Here's how the part is built. I have some questions about the finished solid (model axes, mm). A direction names the side the tool comes from. Round coordinates to 2 decimals unless told otherwise and drop trailing zeros. Order: outer loops, then holes, each group sorted by start corner. A loop starts at its lowest first (then second) coordinate and runs counter-clockwise, first axis right, second up. Notation, with made-up numbers: (72, 52) - (114, 52) arc R14 cw to (114, 72) - close; hole circle Ø1 at (-24, 66). An arc over 180 degrees is marked (long way). Answer as a JSON object with one key per item and string values.
```python
from build123d import *

# Parameters (mm, degrees)
SKETCH1_R           = 7.874
BOSS_EXTRUDE1_DEPTH = 65.024
SKETCH2_R           = 12.7
BOSS_EXTRUDE2_DEPTH = 6.35
CHAMFER1_SIZE       = 2.54


with BuildPart() as part:
    # Sketch1 → Boss-Extrude1 (new body)
    with BuildSketch(Plane.XY):
        Circle(SKETCH1_R)
    extrude(amount=-BOSS_EXTRUDE1_DEPTH)

    # Sketch2 → Boss-Extrude2 (add)
    with BuildSketch(Plane.XY):
        Circle(SKETCH2_R)
    extrude(amount=-BOSS_EXTRUDE2_DEPTH)

    # Chamfer1
    chamfer1_edges = [part.edges().sort_by_distance(p)[0] for p in [
        (-12.7, 0, 0),
    ]]
    chamfer(chamfer1_edges, length=CHAMFER1_SIZE)


solid = part.part
```
1. Imagine slicing it at C-C (z = -50). List the corners of the cut face in (x, y) for me.
Responses:
{"outline": "circle Ø15.75 at (0, 0)"}
2. If I drill on L1, parallel to Z at x = -9.5, y = -5; L2, parallel to X at y = 2, z = -44.5; L3, parallel to Y at x = 0.75, z = -12.5, over which ranges is the centre line in solid material (lowest first)? Write a range as [from, to].
Responses:
{"L1": "[-6.35, -0.58]", "L2": "[-7.62, 7.62]", "L3": "[-7.84, 7.84]"}
3. Imagine slicing it at A-A (x = 0). List the corners of the cut face in (y, z) for me.
Responses:
{"outline": "(-12.7, -6.35) - (-7.87, -6.35) - (-7.87, -65.02) - (7.87, -65.02) - (7.87, -6.35) - (12.7, -6.35) - (12.7, -2.54) - (10.16, 0) - (-10.16, 0) - (-12.7, -2.54) - close"}
4. For faces 1 (the face through (-0.2, -8.3, -6.35)), 2 (the face through (0, 0, -65.024)), which set-ups out of +Z, -Z, +X, -X, +Y, -Y let a thin tool reach every point of the face, with its end or its side?
Responses:
{"face 1": "-Z", "face 2": "-Z, +X, -X, +Y, -Y"}
5. For P1, Ø5, axis at x = -1.5, z = -9, coming from the +Y side; P2, Ø6, axis at y = 6, z = -50, coming from the -X side; P3, Ø8, axis at y = -2, z = -16.5, coming from the +X side, each with a flat end and sliding along its axis, tell me the tip position at first contact or that it passes through.
Responses:
{"P1": "y = 7.87", "P2": "x = -7.28", "P3": "x = 7.87"}
